from build123d import *

# Parameters (mm, degrees)
SKETCH_1_R      = 3.543825796
SKETCH_1_R_2    = 1.357591064
SKETCH_1_W      = 5.3728
SKETCH_1_H      = 3.0001
SKETCH_1_W_2    = 7.9992
EXTRUDE_1_DEPTH = 3


with BuildPart() as part:
    # 草图1 → 凸台-拉伸1 (new body)
    with BuildSketch(Plane.XY.offset(3)):
        with BuildLine():
            Line((-49.343510787, 0), (30.618171933, 0))
            ThreePointArc((30.618171933, 0), (36.618171933, 6), (30.618171933, 12))
            Line((30.618171933, 12), (-49.343510787, 12))
            ThreePointArc((-49.343510787, 12), (-55.343510787, 6), (-49.343510787, 0))
        make_face()
        with Locations((-49.343510787, 6)):
            Circle(SKETCH_1_R, mode=Mode.SUBTRACT)
        with Locations((-13.375343302, 6.0002)):
            Circle(SKETCH_1_R_2, mode=Mode.SUBTRACT)
        with Locations((30.611606698, 6.0001)):
            Circle(SKETCH_1_R_2, mode=Mode.SUBTRACT)
        with Locations((-23.691393302, 5.99945)):
            Rectangle(SKETCH_1_W, SKETCH_1_H, mode=Mode.SUBTRACT)
        with BuildLine():
            Line((-39.352347519, 6.934252935), (-34.404739086, 6.934252935))
            ThreePointArc((-34.404739086, 6.934252935), (-33.487662618, 6.017176468), (-34.404739086, 5.1001))
            Line((-34.404739086, 5.1001), (-39.352347519, 5.1001))
            ThreePointArc((-39.352347519, 5.1001), (-40.269423986, 6.017176468), (-39.352347519, 6.934252935))
        make_face(mode=Mode.SUBTRACT)
        with Locations((16.621706698, 5.99945)):
            Rectangle(SKETCH_1_W_2, SKETCH_1_H, mode=Mode.SUBTRACT)
    extrude(amount=-EXTRUDE_1_DEPTH)


solid = part.part
Verification items for the finished model (mm, model axes). A direction names the side the tool comes from. Coordinates: 2 decimals unless noted, no trailing zeros. Order: outer loops, then holes, each group sorted by start corner. A loop starts at its lowest first (then second) coordinate and runs counter-clockwise, first axis right, second up. Notation, with made-up numbers: M -30.75,-26.75 L 1.25,-26.75 A15 ccw 1.25,-4.75 Z; hole C -17.75,70.25 d3. An arc over 180 degrees is marked long. Return JSON: item names as keys, results as strings.
1) Thickness scan on L1, parallel to Y at x = -34.5, z = 1.4; L2, parallel to Y at x = 14.5, z = 1.7; L3, parallel to X at y = 3.25, z = 1. Record the ranges inside material, lowest first. Write a range as [from, to].
Answer list:
{"L1": "[0, 5.1], [6.93, 12]", "L2": "[0, 4.5], [7.5, 12]", "L3": "[-54.68, -51.58], [-47.11, 35.95]"}
2) Release check for a two-part mould opening along X. For faces 1 (the flat face through (-10, 6, 0)), 2 (the cylindrical face through (-55.342, 6.132, 1.521)), 3 (the flat face through (-24, 7.5, 2)) record: +X half, -X half, draft (parallel to the pull), parting line (faces both ways), or undercut.
Answer list:
{"face 1": "draft", "face 2": "-X half", "face 3": "undercut"}
3) Cross-section at A-A, the plane y = 3.25. Record the boundary of the cut face in (x, z).
Answer list:
{"outline": "M -54.68,0 L -51.58,0 L -51.58,3 L -54.68,3 Z; M -47.11,0 L 35.95,0 L 35.95,3 L -47.11,3 Z"}
4) Cross-section at B-B, the plane z = 0.7. Record the boundary of the cut face in (x, y) (1 decimal).
Answer list:
{"outline": "M -49.3,0 L 30.6,0 A6 ccw 30.6,12 L -49.3,12 A6 ccw Z; hole C -49.3,6 d7.1; hole M -39.4,5.1 L -34.4,5.1 A0.9 ccw -34.4,6.9 L -39.4,6.9 A0.9 ccw Z; hole M -26.4,4.5 L -21,4.5 L -21,7.5 L -26.4,7.5 Z; hole C -13.4,6 d2.7; hole M 12.6,4.5 L 20.6,4.5 L 20.6,7.5 L 12.6,7.5 Z; hole C 30.6,6 d2.7"}
5) Gauge pin test, flat end, axial feed: pin 1 (1 mm diameter, centred on y = 9, z = 1, fed in from -X). Record the tip position at first contact, or that the pin passes through.
Answer list:
{"pin 1": "x = -54.8"}
6) Access from +Z, -Z, +X, -X, +Y, -Y to the whole of each face (thin tool, end or side, straight path). Record for faces 4 (the flat face through (-10, 0, 2)), 5 (the flat face through (-24, 4.499, 2)).
Answer list:
{"face 4": "+Z, -Z, +X, -X, -Y", "face 5": "+Z, -Z"}
7) Cross-section at C-C, the plane y = 8.5. Record the boundary of the cut face in (x, z).
Answer list:
{"outline": "M -54.8,0 L -51.86,0 L -51.86,3 L -54.8,3 Z; M -46.83,0 L 36.07,0 L 36.07,3 L -46.83,3 Z"}
